Part print with two shaded views. Sizes in mm from the minimum x, y, z corner. Coordinates: 2 decimals unless noted, no trailing zeros. Loops run counter-clockwise (first coordinate to the right, second up) from the corner with the lowest first, then second, coordinate; pieces in that order, holes last. Notation, with made-up numbers: (16.25, 4) -> (56.25, 4) arc R31 ccw to (56.25, 32) -> close; hole circle Ø2 at (39.25, -23.75). An arc over 180 degrees is marked (long way). Return JSON: item names as keys, results as strings. Group by question number.
(1) Saw through at D-D on y = 4. Write the cut outline in (x, z), then the cut area to 3 significant figures.
(2) Saw through at A-A on y = 25. Write the cut outline in (x, z).
(3) Mould opens along Y. For the marked faces 1, 2 and 3 say: pulls with the +Y half, pulls with the -Y half, needs draft (parallel to the pull), parting line crosses it, or undercut.
(4) Saw through at B-B on x = 8.5. Write the cut outline in (y, z).
(5) Saw through at C-C on y = 37.5. Write the cut outline in (x, z), then the cut area to 3 significant figures.
(6) Probe L1, parallel to Y at x = 7.75, z = 80; L2, parallel to Z at x = 5, y = 18.5; L3, parallel to Z at x = 1.5, y = 21. List the from-to ranges inside material, lowest first.
(7) Flat gauge pin, fed straight in: pin 1 Ø3 at (x, y) = (1, 25) entering from +Z. Where does the tip first touch, or does it go through?
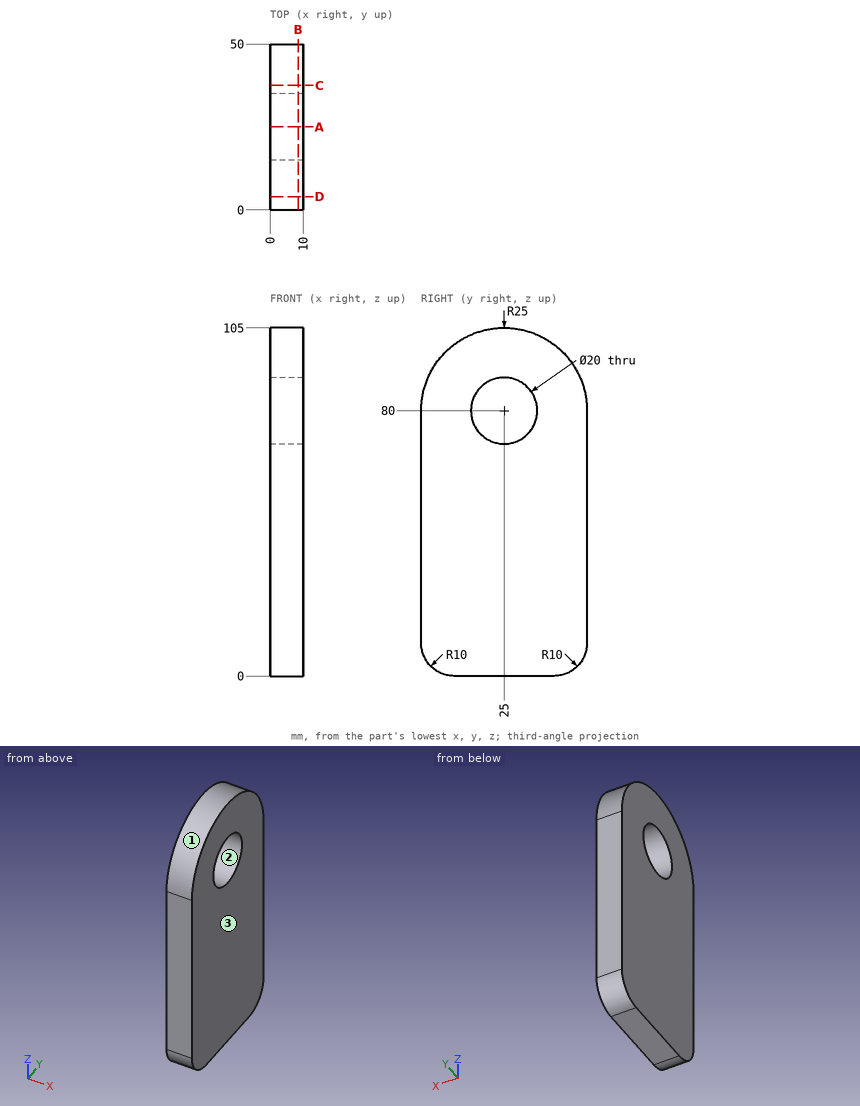
Geometry results:
{
 "1": {"outline": "(0, 2) -> (10, 2) -> (10, 93.56) -> (0, 93.56) -> close", "area": "916 mm²"},
 "2": {"outline": "(0, 0) -> (10, 0) -> (10, 70) -> (0, 70) -> close; (0, 90) -> (10, 90) -> (10, 105) -> (0, 105) -> close"},
 "3": {"face 1": "parting line crosses it", "face 2": "undercut", "face 3": "needs draft"},
 "4": {"outline": "(0, 10) arc R10 ccw to (10, 0) -> (40, 0) arc R10 ccw to (50, 10) -> (50, 80) arc R25 ccw to (0, 80) -> close; hole circle Ø20 at (25, 80)"},
 "5": {"outline": "(0, 0) -> (10, 0) -> (10, 101.65) -> (0, 101.65) -> close", "area": "1,020 mm²"},
 "6": {"L1": "0 to 15, 35 to 50", "L2": "0 to 72.4, 87.6 to 104.14", "L3": "0 to 70.83, 89.17 to 104.68"},
 "7": {"pin 1": "z = 105"}
}
